```python
from build123d import *

# Parameters (mm, degrees)
BOSS_EXTRUDE1_DEPTH = 3
CUT_EXTRUDE1_DEPTH  = 4


with BuildPart() as part:
    # Sketch1 → Boss-Extrude1 (new body)
    with BuildSketch(Plane.XY):
        with BuildLine():
            Line((60, 65.779396594), (60, 0))
            Line((60, 0), (-60, 0))
            Line((-60, 0), (-60, 65.779396594))
            ThreePointArc((-60, 65.779396594), (-24.19023261, 103.91162188), (-29.909652169, 155.908682236))
            Line((-29.909652169, 155.908682236), (-29.909652169, 180.455528653))
            Line((-29.909652169, 180.455528653), (29.909652169, 180.455528653))
            Line((29.909652169, 180.455528653), (29.909652169, 155.908682236))
            ThreePointArc((29.909652169, 155.908682236), (24.19023261, 103.91162188), (60, 65.779396594))
        make_face()
    extrude(amount=BOSS_EXTRUDE1_DEPTH)

    # Sketch2 → Cut-Extrude1 (cut, through all)
    with BuildSketch(Plane.XY.offset(3)):
        with BuildLine():
            Line((-60, 60), (-60, -14.155296416))
            Line((-60, -14.155296416), (60, -14.155296416))
            Line((60, -14.155296416), (60, 60))
            ThreePointArc((60, 60), (0, 0), (-60, 60))
        make_face()
    extrude(amount=-CUT_EXTRUDE1_DEPTH, mode=Mode.SUBTRACT)


solid = part.part
```
Work out the finished part from the listing and answer in its coordinate system (mm). Give positions to 0.01 mm unless a question says otherwise; leave off trailing zeros. Loops run counter-clockwise (first coordinate to the right, second up) from the corner with the lowest first, then second, coordinate; pieces in that order, holes last. Notation, with made-up numbers: (6.25, 76) -> (63.25, 76) arc R9 ccw to (63.25, 90) -> close; hole circle Ø4 at (41.5, 10). An arc over 180 degrees is marked (long way). Put each result on its own line as item: value. Start each with the question number.
Item 1: The part is cut by section B-B (y = 75). Give the vertices of the cut face in (x, z), then the cut area to 3 significant figures.
Item 2: Find the intervals of material crossed by L1, parallel to X at y = 161.5, z = 2.7; L2, parallel to X at y = 32.5, z = 0.85; L3, parallel to Y at x = -47, z = 0.6, in increasing order. Write a range as [from, to].
Item 3: The part is cut by section C-C (x = 50.5). Give the vertices of the cut face in (y, z).
Item 4: Each of these flat-tipped pins is pushed along its axis until it touches: P1, Ø1.5, axis at y = 163.5, z = 2, coming from the -X side; P2, Ø1.5, axis at y = 89, z = 2, coming from the -X side; P3, Ø0.9, axis at y = 170, z = 1, coming from the +X side. Where does it stop, or does it pass through?
Item 5: The part is cut by section A-A (z = 2.1). Give the vertices of the cut face in (x, y), then the cut area to 3 significant figures.
Item 6: The mould has two halves that part along Y. Classify faces 1 (the face through (23.955, 104.63, 1.479)), 2 (the face through (1, 91, 0)), 3 (the face through (1.319, 0.015, 1.521)): released by +Y, released by -Y, zero draft, split by the parting line, or undercut.
Answers below:
1. outline: (-44.3, 0) -> (44.3, 0) -> (44.3, 3) -> (-44.3, 3) -> close
1. area: 266 mm2
2. L1: [-29.91, 29.91]
2. L2: [-53.33, 53.33]
2. L3: [22.7, 72.95]
3. outline: (27.6, 0) -> (70.61, 0) -> (70.61, 3) -> (27.6, 3) -> close
4. P1: x = -29.91
4. P2: x = -32
4. P3: x = 29.91
5. outline: (-60, 60) arc R60 ccw to (60, 60) -> (60, 65.78) arc R62.5 cw to (29.91, 155.91) -> (29.91, 180.46) -> (-29.91, 180.46) -> (-29.91, 155.91) arc R62.5 cw to (-60, 65.78) -> close
5. area: 13,000 mm2
6. face 1: undercut
6. face 2: zero draft
6. face 3: released by -Y
